The listing builds one solid part. Answer for the finished solid, in the listing's coordinates (mm). A direction names the side the tool comes from. Coordinates: 2 decimals unless noted, no trailing zeros. Order: outer loops, then holes, each group sorted by start corner. A loop starts at its lowest first (then second) coordinate and runs counter-clockwise, first axis right, second up.
```python
from build123d import *

# Parameters (mm, degrees)
BOSS_EXTRU_1_DEPTH      = 3
BOSS_EXTRU_2_DEPTH      = 44
BOSS_EXTRU_4_START      = -3
BOSS_EXTRU_4_DEPTH      = 3
BOSS_EXTRU_6_DEPTH      = 16
ESQUISSE10_W            = 71
ESQUISSE10_H            = 3
BOSS_EXTRU_10_DEPTH     = 7
ESQUISSE12_R            = 2
ENL_V_MAT_EXTRU_1_DEPTH = 73.94861205
ESQUISSE13_W            = 12
ESQUISSE13_H            = 3
BOSS_EXTRU_11_DEPTH     = 9.5
ESQUISSE14_W            = 12
ESQUISSE14_H            = 3
BOSS_EXTRU_12_DEPTH     = 9.5
ESQUISSE15_W            = 12
ESQUISSE15_H            = 3
BOSS_EXTRU_13_DEPTH     = 4
ESQUISSE16_W            = 12
ESQUISSE16_H            = 3
BOSS_EXTRU_14_DEPTH     = 4
CONG_7_R                = 1


with BuildPart() as part:
    # Esquisse1 → Boss.-Extru.1 (new body)
    with BuildSketch(Plane.XY):
        with BuildLine():
            Line((-18.5, 0), (-14.5, 0))
            ThreePointArc((-14.5, 0), (0, 14.5), (14.5, 0))
            Line((14.5, 0), (18.5, 0))
            ThreePointArc((18.5, 0), (0, 18.5), (-18.5, 0))
        make_face()
    extrude(amount=BOSS_EXTRU_1_DEPTH)

    # Esquisse3 → Boss.-Extru.2 (add)
    with BuildSketch(Plane.XY.offset(3)):
        with BuildLine():
            Line((-18.5, 0), (-16.25, 0))
            ThreePointArc((-16.25, 0), (0, 16.25), (16.25, 0))
            Line((16.25, 0), (18.5, 0))
            ThreePointArc((18.5, 0), (0, 18.5), (-18.5, 0))
        make_face()
    extrude(amount=BOSS_EXTRU_2_DEPTH)

    # Esquisse4 → Boss.-Extru.4 (add)
    with BuildSketch(Plane.XY.offset(47).offset(BOSS_EXTRU_4_START)):
        with BuildLine():
            Line((9, 0), (18.5, 0))
            ThreePointArc((18.5, 0), (0, 18.5), (-18.5, 0))
            Line((-18.5, 0), (-9, 0))
            Line((-9, 0), (-9, 3.618010503))
            ThreePointArc((-9, 3.618010503), (0, 9.7), (9, 3.618010503))
            Line((9, 3.618010503), (9, 0))
        make_face()
    extrude(amount=BOSS_EXTRU_4_DEPTH)

    # Esquisse6 → Boss.-Extru.6 (add)
    with BuildSketch(Plane.XZ):
        Polygon((14.5, 3), (16.25, 3), (16.25, 44), (9, 44), (9, 47), (18.5, 47), (18.5, 0), (14.5, 0), align=None)
        Polygon((-14.5, 3), (-14.5, 0), (-18.5, 0), (-18.5, 47), (-9, 47), (-9, 44), (-16.25, 44), (-16.25, 3), align=None)
    extrude(amount=BOSS_EXTRU_6_DEPTH)

    # Esquisse10 → Boss.-Extru.10 (add)
    with BuildSketch(Plane(origin=(18.5, 0, 0), x_dir=(0, 0, -1), z_dir=(1, 0, 0))):
        with Locations((-23.5, -14.5)):
            Rectangle(ESQUISSE10_W, ESQUISSE10_H)
    boss_extru_10 = extrude(amount=BOSS_EXTRU_10_DEPTH)

    # Symétrie4: Boss.-Extru.10 across plane
    add(boss_extru_10.mirror(Plane(origin=(0, 0, 0), x_dir=(0, 0, 1), z_dir=(1, 0, 0))))

    # Esquisse12 → Enlèv. mat.-Extru.1 (cut, through all)
    with BuildSketch(Plane.XZ.offset(16)):
        with Locations(Location((21, 54.85, 0), (0, 0, 270))):
            Circle(ESQUISSE12_R)
        with Locations(Location((21, -7.85, 0), (0, 0, 270))):
            Circle(ESQUISSE12_R)
        with Locations(Location((-21, -7.85, 0), (0, 0, 270))):
            Circle(ESQUISSE12_R)
        with Locations(Location((-21, 54.85, 0), (0, 0, 270))):
            Circle(ESQUISSE12_R)
    extrude(amount=-ENL_V_MAT_EXTRU_1_DEPTH, mode=Mode.SUBTRACT)

    # Esquisse13 → Boss.-Extru.11 (add)
    with BuildSketch(Plane(origin=(-18.5, 0, 0), x_dir=(0, 0, -1), z_dir=(1, 0, 0))):
        with Locations((-53, -14.5)):
            Rectangle(ESQUISSE13_W, ESQUISSE13_H)
    extrude(amount=BOSS_EXTRU_11_DEPTH)

    # Esquisse14 → Boss.-Extru.12 (add)
    with BuildSketch(Plane.ZY.offset(-18.5)):
        with Locations((53, -14.5)):
            Rectangle(ESQUISSE14_W, ESQUISSE14_H)
    extrude(amount=BOSS_EXTRU_12_DEPTH)

    # Esquisse15 → Boss.-Extru.13 (add)
    with BuildSketch(Plane.ZY.offset(-18.5)):
        with Locations((-6, -14.5)):
            Rectangle(ESQUISSE15_W, ESQUISSE15_H)
    extrude(amount=BOSS_EXTRU_13_DEPTH)

    # Esquisse16 → Boss.-Extru.14 (add)
    with BuildSketch(Plane(origin=(-18.5, 0, 0), x_dir=(0, 0, -1), z_dir=(1, 0, 0))):
        with Locations((6, -14.5)):
            Rectangle(ESQUISSE16_W, ESQUISSE16_H)
    extrude(amount=BOSS_EXTRU_14_DEPTH)

    # Congé7
    cong_7_edges = [part.edges().sort_by_distance(p)[0] for p in [
        (-18.5, -6.5, 0),
        (-18.5, -6.5, 47),
        (-18.5, -13, 23.5),
        (-20, -13, -12),
        (-25.5, -13, 23.5),
        (-17.25, -13, 59),
        (-13.75, -13, 47),
        (13.75, -13, 47),
        (0, 18.5, 47),
        (16.5, -13, 0),
        (-16.5, -13, 0),
        (0, 18.5, 0),
        (18.5, -6.5, 47),
        (18.5, -6.5, 0),
        (18.5, -13, 23.5),
        (20, -13, -12),
        (17.25, -13, 59),
        (25.5, -13, 23.5),
    ]]
    fillet(cong_7_edges, radius=CONG_7_R)


solid = part.part
```
(1) Consider line 1 (X direction, y = -15.35, z = -7.85); line 2 (X direction, y = -15.15, z = 54.85); line 3 (X direction, y = -4, z = 9). Determine where each line is inside the solid, lowest interval first.
(2) Find section A-A (z = 54.85). Write down the section's boundary in (x, y), and give its area (3 significant figures).
(3) For faces 1 (the face through (-9, -9.8, 46.5)), 2 (the face through (-14.5, -11, 1)), 3 (the face through (18.5, -6, 24)), 4 (the face through (-7, 8, 44)), determine the directions among +Z, -Z, +X, -X, +Y, -Y from which every point of the face is accessible in a straight line to the end or side of a thin tool.
(4) Find section C-C (z = -5). Write down the section's boundary in (x, y).
(5) The mould has two halves that part along X. Classify faces 5 (the face through (17, -15, 59)), 6 (the face through (25.5, -15, 24)), 7 (the face through (-10, 11, 3)), 8 (the face through (14.5, -11.4, 0.4)): released by +X, released by -X, zero draft, split by the parting line, or undercut.
(6) Find section B-B (x = 21). Write down the section's boundary in (y, z).
(7) Each of these flat-tipped pins is pushed along its axis until it touches: pin 1 Ø13 at (y, z) = (-5, 29) entering from +X; pin 2 Ø8 at (y, z) = (7, 45.5) entering from +X; pin 3 Ø4.5 at (y, z) = (-6, -4) entering from -X; pin 4 Ø6 at (x, y) = (8.5, 11.5) entering from +Z. Where does it stop, or does it pass through?
(8) Find section D-D (x = 0). Write down the section's boundary in (y, z).
Findings below:
1. line 1: x = -25.5 to -23, -19 to -14.5, 14.5 to 19, 23 to 25.5
1. line 2: x = -25.5 to -23, -19 to -9, 9 to 19, 23 to 25.5
1. line 3: x = -18.5 to -16.25, 16.25 to 18.5
2. outline: (-25.5, -16) - (-23, -16) - (-23, -13) - (-24.5, -13) arc R1 ccw to (-25.5, -14) - close; (-19, -16) - (-9, -16) - (-9, -13) - (-19, -13) - close; (9, -16) - (19, -16) - (19, -13) - (9, -13) - close; (23, -16) - (25.5, -16) - (25.5, -14) arc R1 ccw to (24.5, -13) - (23, -13) - close
2. area: 74.6 mm2
3. face 1: +Z, -Z, -Y
3. face 2: -Z, -Y
3. face 3: +Z, -Z, +X, +Y
3. face 4: -Y
4. outline: (-25.5, -16) - (-14.5, -16) - (-14.5, -13) - (-24.5, -13) arc R1 ccw to (-25.5, -14) - close; (14.5, -16) - (25.5, -16) - (25.5, -14) arc R1 ccw to (24.5, -13) - (14.5, -13) - close
5. face 5: zero draft
5. face 6: released by +X
5. face 7: undercut
5. face 8: undercut
6. outline: (-16, -12) - (-14, -12) arc R1 ccw to (-13, -11) - (-13, -9.85) - (-16, -9.85) - close; (-16, -5.85) - (-13, -5.85) - (-13, 52.85) - (-16, 52.85) - close; (-16, 56.85) - (-13, 56.85) - (-13, 58) arc R1 ccw to (-14, 59) - (-16, 59) - close
7. pin 1: stops at x = 18.5
7. pin 2: stops at x = 18.26
7. pin 3: passes through
7. pin 4: stops at z = 47
8. outline: (9.7, 44) - (16.25, 44) - (16.25, 3) - (14.5, 3) - (14.5, 0) - (17.5, 0) arc R1 ccw to (18.5, 1) - (18.5, 46) arc R1 ccw to (17.5, 47) - (9.7, 47) - close
